from build123d import *

# Parameters (mm, degrees)
SKETCH2_W            = 218
SKETCH2_H            = 30
BOSS_EXTRUDE1_DEPTH  = 5
FILLET1_R            = 20
SKETCH3_R            = 10
CUT_EXTRUDE1_DEPTH   = 4
SKETCH3_3_R          = 10
CUT_EXTRUDE2_DEPTH   = 4
CHAMFER1_SIZE        = 3
SKETCH6_R            = 5
CUT_EXTRUDE3_DEPTH   = 119.749210232
BOSS_EXTRUDE2_DEPTH  = 20
SKETCH8_W            = 30
SKETCH8_H            = 21.4
BOSS_EXTRUDE3_DEPTH  = 3
SKETCH10_W           = 30
SKETCH10_H           = 21.4
CUT_EXTRUDE4_DEPTH   = 3
CUT_EXTRUDE5_DEPTH   = 40
FILLET2_R            = 10
FILLET2_OF_MIRROR1_R = 10


with BuildPart() as part:
    # Sketch2 → Boss-Extrude1 (new, symmetric)
    with BuildSketch(Plane.XY):
        Rectangle(SKETCH2_W, SKETCH2_H)
    extrude(amount=BOSS_EXTRUDE1_DEPTH, both=True)

    # Fillet1
    fillet1_edges = [part.edges().sort_by_distance(p)[0] for p in [
        (109, -15, 0),
        (-109, -15, 0),
    ]]
    fillet(fillet1_edges, radius=FILLET1_R)

    # Sketch3 → Cut-Extrude1 (cut)
    with BuildSketch(Plane.XY.offset(5)):
        with Locations((-91, 2)):
            Circle(SKETCH3_R)
    extrude(amount=-CUT_EXTRUDE1_DEPTH, mode=Mode.SUBTRACT)

    # Sketch3<3> → Cut-Extrude2 (cut)
    with BuildSketch(Plane.XY.offset(5)):
        with Locations((-91, 2)):
            Circle(SKETCH3_3_R)
        with Locations((-31, 2)):
            Circle(SKETCH3_3_R)
    extrude(amount=-CUT_EXTRUDE2_DEPTH, mode=Mode.SUBTRACT)

    # Chamfer1
    chamfer1_edges = [part.edges().sort_by_distance(p)[0] for p in [
        (-101, 2, 5),
        (-41, 2, 5),
    ]]
    chamfer(chamfer1_edges, length=CHAMFER1_SIZE - 0.0001)  # a hair under: the kernel refuses the full size

    # Sketch5 → Revolve1 (revolve)
    with BuildSketch(Plane(origin=(-61.85, 0, 0), x_dir=(0, 0, -1), z_dir=(1, 0, 0)), mode=Mode.PRIVATE) as revolve1_sk:
        Polygon((-20.498711306, 18.495190528), (-24.248711306, 12), (10.392304845, -8), (14.142304845, -1.504809472), align=None)
    revolve(revolve1_sk.sketch.rotate(Axis((-61.85, 12, 24.248711306), (0, -0.49999999999999767, -0.86602540378444)), 180), axis=Axis((-61.85, 12, 24.248711306), (0, -0.49999999999999767, -0.86602540378444)))

    # Sketch6 → Cut-Extrude3 (cut, through all)
    with BuildSketch(Plane(origin=(0, 13.5, 23.382685902), x_dir=(1, 0, 0), z_dir=(0, 0.4999999999999978, 0.86602540378444))):
        with Locations(Location((-61.85, -1.732050808, 0), (0, 0, 270))):
            Circle(SKETCH6_R)
    extrude(amount=-CUT_EXTRUDE3_DEPTH, mode=Mode.SUBTRACT)

    # Sketch7 → Boss-Extrude2 (add, symmetric)
    with BuildSketch(Plane(origin=(0, 0, 0), x_dir=(0, 0, -1), z_dir=(1, 0, 0))):
        Polygon((5, -15), (-5, -15), (-33.867513459, -65), (-91.641016151, -65), (-91.641016151, -75), (-29.641016151, -75), align=None)
    extrude(amount=BOSS_EXTRUDE2_DEPTH, both=True)

    # Sketch8 → Boss-Extrude3 (add)
    with BuildSketch(Plane(origin=(0, -1.584936491, -2.745190528), x_dir=(1, 0, 0), z_dir=(0, 0.4999999999999978, 0.86602540378444))):
        with Locations((0, -31.190381057)):
            Rectangle(SKETCH8_W, SKETCH8_H)
    extrude(amount=BOSS_EXTRUDE3_DEPTH)

    # Sketch10 → Cut-Extrude4 (cut)
    with BuildSketch(Plane(origin=(0, -1.584936491, -2.745190528), x_dir=(1, 0, 0), z_dir=(0, 0.499999999999998, 0.8660254037844398))):
        with Locations((0, -57.525407976)):
            Rectangle(SKETCH10_W, SKETCH10_H)
    extrude(amount=-CUT_EXTRUDE4_DEPTH, mode=Mode.SUBTRACT)

    # Sketch11 → Revolve2 (revolve)
    with BuildSketch(Plane(origin=(0, 0, 0), x_dir=(0, 0, -1), z_dir=(1, 0, 0)), mode=Mode.PRIVATE) as revolve2_sk:
        with BuildLine():
            Line((-61.641016151, -23.08118878), (-61.641016151, -85))
            Line((-61.641016151, -85), (-54.141016151, -85))
            Line((-54.141016151, -85), (-54.141016151, -75))
            Line((-54.141016151, -75), (-56.641016151, -75))
            Line((-56.641016151, -75), (-56.641016151, -63))
            ThreePointArc((-56.641016151, -63), (-57.519695808, -60.878679656), (-59.641016151, -60))
            Line((-59.641016151, -60), (-59.641016151, -36.58459552))
            ThreePointArc((-59.641016151, -36.58459552), (-54.92395374, -28.986133621), (-61.641016151, -23.08118878))
        make_face()
    revolve(revolve2_sk.sketch.rotate(Axis((0, -23.08118878, 61.641016151), (0, -1, 0)), 180), axis=Axis((0, -23.08118878, 61.641016151), (0, -1, 0)))

    # Sketch12 → Cut-Extrude5 (cut)
    with BuildSketch(Plane(origin=(0, 15, 0), x_dir=(1, 0, 0), z_dir=(0, 1, 0))):
        Polygon((-109, -5), (-109, 5), (-105.52, 5), align=None)
    cut_extrude5 = extrude(amount=-CUT_EXTRUDE5_DEPTH, mode=Mode.SUBTRACT)

    # Fillet2
    fillet2_edges = [part.edges().sort_by_distance(p)[0] for p in [
        (-107.26, 15, 0),
    ]]
    fillet(fillet2_edges, radius=FILLET2_R)

    # Mirror1: Cut-Extrude5 across plane
    add(cut_extrude5.mirror(Plane(origin=(0, 0, 0), x_dir=(0, 0, 1), z_dir=(1, 0, 0))), mode=Mode.SUBTRACT)

    # Fillet2 of Mirror1
    fillet2_of_mirror1_edges = [part.edges().sort_by_distance(p)[0] for p in [
        (107.26, 15, 0),
    ]]
    fillet(fillet2_of_mirror1_edges, radius=FILLET2_OF_MIRROR1_R)


solid = part.part
Design review of the part built by this model. Coordinates are the model's own, in mm. A direction names the side the tool comes from. Coordinates: 2 decimals unless noted, no trailing zeros. Write each loop counter-clockwise with the first axis right and the second up, starting at its lowest first coordinate (ties: lowest second). Pieces come first, ordered by that corner, then holes. Notation, with made-up numbers: (-8.75, 36) - (11.25, 36) arc R20 ccw to (11.25, 67) - close; hole circle Ø7 at (-22, -2.5). An arc over 180 degrees is marked (long way). One line per item, written item: value.
1) Mouldability with a two-part tool opening along Z and no side actions: class faces 5 (the face through (-100.99, 2.44, 1.51)), 6 (the face through (106.85, 0.69, -1.18)), 7 (the face through (-0.6, -48.13, 63.55)) as +Z half, -Z half, draft (parallel to the pull), parting line (faces both ways), or undercut.
Answer sheet:
face 5: draft
face 6: -Z half
face 7: undercut
2) For faces 1 (the face through (-2.253, -79.93, 68.795)), 2 (the face through (-40.99, 2.44, 1.51)), 3 (the face through (-0.21, -26.967, 15.373)), 4 (the face through (54, -15, 0)), list the 3-axis set-ups (+Z, -Z, +X, -X, +Y, -Y) from which the entire face can be reached by the end or side of a thin tool; tool diameter is ignored.
Answer sheet:
face 1: -Y
face 2: +Z
face 3: +X, -X, +Y
face 4: +Z, -Z, +X, -Y
3) Add section B-B (z = 72). State the section outline as (x, y) points, plus the area to 3 significant figures.
Answer sheet:
outline: (-20, -75) - (20, -75) - (20, -65) - (-20, -65) - close
area: 400 mm2
4) Add section C-C (y = -67.5). State the section outline as (x, z) points, plus the area to 3 significant figures.
Answer sheet:
outline: (-20, 25.31) - (20, 25.31) - (20, 91.64) - (-20, 91.64) - close
area: 2,650 mm2
5) Insertion check: pin 1 (3 mm diameter, centred on x = 51.5, z = 2, fed in from -Y); pin 2 (1 mm diameter, centred on y = -57.5, z = 25, fed in from -X); pin 3 (6 mm diameter, centred on x = -94, y = 7, fed in from +Z). Each pin has a flat end and moves straight along its axis. Give the tip position at first contact, or say it passes through.
Answer sheet:
pin 1: stops at y = -15
pin 2: stops at x = -20
pin 3: stops at z = 1
6) To check wall thickness, follow probe 1 along Y at (x, z) = (-31, 1.4); probe 2 along Z at (x, y) = (87, -3); probe 3 along X at (y, z) = (-74, 69.5). State the ranges of each line that lie inside material, in increasing order.
Answer sheet:
probe 1: y = -15 to -8, 12 to 15
probe 2: z = -5 to 5
probe 3: x = -20 to 20
